Input: part model. Units: mm. Frame: model coordinates. A direction names the side the tool comes from. Coordinates: 2 decimals unless noted, no trailing zeros. Loops run counter-clockwise (first coordinate to the right, second up) from the corner with the lowest first, then second, coordinate; pieces in that order, holes last. Notation, with made-up numbers: (-17, 17) - (-5, 17) arc R20 ccw to (-5, 40) - close; hole circle Ø8 at (22.25, 9.25). An arc over 180 degrees is marked (long way). Use one line per item in the form item = value.
from build123d import *

# Parameters (mm, degrees)
SKETCH1_R           = 2.5
SKETCH1_R_2         = 3.5
SKETCH1_W           = 71.85
SKETCH1_H           = 24.6
SKETCH1_W_2         = 12.2
SKETCH1_H_2         = 12.2
SKETCH1_W_3         = 10.2
SKETCH1_H_3         = 14.85
BOSS_EXTRUDE1_DEPTH = 3
FILLET1_R           = 2
FILLET2_R           = 3
BOSS_EXTRUDE2_START = -10
BOSS_EXTRUDE2_DEPTH = 10
BOSS_EXTRUDE3_START = -10
BOSS_EXTRUDE3_DEPTH = 10


with BuildPart() as part:
    # Sketch1 → Boss-Extrude1 (new body)
    with BuildSketch(Plane.XY):
        Polygon((0, 0), (-115, 0), (-115, -51), (-143, -51), (-143, -99), (-115, -99), (0, -99), (28, -99), (28, -51), (0, -51), align=None)
        with Locations((-57.5, -10.395373235)):
            Circle(SKETCH1_R, mode=Mode.SUBTRACT)
        with Locations((-19.5, -32.493549158)):
            Circle(SKETCH1_R_2, mode=Mode.SUBTRACT)
        with Locations((-45.247302804, -78.7)):
            Rectangle(SKETCH1_W, SKETCH1_H, mode=Mode.SUBTRACT)
        with Locations((-98.6, -53.697377152)):
            Rectangle(SKETCH1_W_2, SKETCH1_H_2, mode=Mode.SUBTRACT)
        with Locations((-95.5, -32.493549158)):
            Rectangle(SKETCH1_W_3, SKETCH1_H_3, mode=Mode.SUBTRACT)
        with Locations((-16.4, -53.697377152)):
            Rectangle(SKETCH1_W_2, SKETCH1_H_2, mode=Mode.SUBTRACT)
    extrude(amount=BOSS_EXTRUDE1_DEPTH)

    # Fillet1
    fillet1_edges = [part.edges().sort_by_distance(p)[0] for p in [
        (-115, -25.5, 3),
        (-129, -51, 3),
        (-143, -75, 3),
        (-57.5, -99, 3),
        (28, -75, 3),
        (14, -51, 3),
        (0, -25.5, 3),
        (-57.5, 0, 3),
    ]]
    fillet(fillet1_edges, radius=FILLET1_R)

    # Fillet2
    # the kernel refuses this fillet: 3 mm, written as the material it takes off along each edge
    with BuildSketch(Plane(origin=(-140, -54, 3), x_dir=(0, 1, 0), z_dir=(1, 0, 0))) as fillet2_piece_1:
        with BuildLine():
            CenterArc((1, -2), 2, 0, 90)
            Line((3, -2), (3, 0))
            Line((3, 0), (1, 0))
        make_face()
    revolve(axis=Axis((-140, -54, 3), (0, 0, 1)), revolution_arc=90, mode=Mode.SUBTRACT)
    with BuildSketch(Plane(origin=(-140, -96, 3), x_dir=(-1, 0, 0), z_dir=(0, 1, 0))) as fillet2_piece_2:
        with BuildLine():
            CenterArc((1, -2), 2, 0, 90)
            Line((3, -2), (3, 0))
            Line((3, 0), (1, 0))
        make_face()
    revolve(axis=Axis((-140, -96, 3), (0, 0, 1)), revolution_arc=90, mode=Mode.SUBTRACT)
    with BuildSketch(Plane(origin=(-112, -3, 3), x_dir=(0, 1, 0), z_dir=(1, 0, 0))) as fillet2_piece_3:
        with BuildLine():
            CenterArc((1, -2), 2, 0, 90)
            Line((3, -2), (3, 0))
            Line((3, 0), (1, 0))
        make_face()
    revolve(axis=Axis((-112, -3, 3), (0, 0, 1)), revolution_arc=90, mode=Mode.SUBTRACT)
    with BuildSketch(Plane(origin=(25, -96, 3), x_dir=(0, -1, 0), z_dir=(-1, 0, 0))) as fillet2_piece_4:
        with BuildLine():
            CenterArc((1, -2), 2, 0, 90)
            Line((3, -2), (3, 0))
            Line((3, 0), (1, 0))
        make_face()
    revolve(axis=Axis((25, -96, 3), (0, 0, 1)), revolution_arc=90, mode=Mode.SUBTRACT)
    with BuildSketch(Plane(origin=(-3, -3, 3), x_dir=(1, 0, 0), z_dir=(0, -1, 0))) as fillet2_piece_5:
        with BuildLine():
            CenterArc((1, -2), 2, 0, 90)
            Line((3, -2), (3, 0))
            Line((3, 0), (1, 0))
        make_face()
    revolve(axis=Axis((-3, -3, 3), (0, 0, 1)), revolution_arc=90, mode=Mode.SUBTRACT)
    with BuildSketch(Plane(origin=(25, -54, 3), x_dir=(1, 0, 0), z_dir=(0, -1, 0))) as fillet2_piece_6:
        with BuildLine():
            CenterArc((1, -2), 2, 0, 90)
            Line((3, -2), (3, 0))
            Line((3, 0), (1, 0))
        make_face()
    revolve(axis=Axis((25, -54, 3), (0, 0, 1)), revolution_arc=90, mode=Mode.SUBTRACT)
    with BuildSketch(Plane(origin=(28, -51, -7.5), x_dir=(-1, 0, 0), z_dir=(0, 0, 1)), Plane(origin=(0, 0, -7.5), x_dir=(-1, 0, 0), z_dir=(0, 0, 1))) as fillet2_piece_7:
        with BuildLine():
            CenterArc((FILLET2_R, FILLET2_R), FILLET2_R, 180, 90)
            Line((0, FILLET2_R), (0, 0))
            Line((0, 0), (FILLET2_R, 0))
        make_face()
    extrude(amount=10.5, mode=Mode.SUBTRACT)
    with BuildSketch(Plane(origin=(-115, 0, -7.5), x_dir=(1, 0, 0), z_dir=(0, 0, 1)), Plane(origin=(-143, -51, -7.5), x_dir=(1, 0, 0), z_dir=(0, 0, 1)), Plane(origin=(28, -99, -7.5), x_dir=(-1, 0, 0), z_dir=(0, 0, 1)), Plane(origin=(-143, -99, -7.5), x_dir=(0, 1, 0), z_dir=(0, 0, 1))) as fillet2_piece_8:
        with BuildLine():
            CenterArc((FILLET2_R, -FILLET2_R), FILLET2_R, 90, 90)
            Line((0, -FILLET2_R), (0, 0))
            Line((0, 0), (FILLET2_R, 0))
        make_face()
    extrude(amount=10.5, mode=Mode.SUBTRACT)

    # Sketch3 → Boss-Extrude2 (add)
    with BuildSketch(Plane(origin=(0, -60, 0), x_dir=(1, 0, 0), z_dir=(0, 1, 0)).offset(BOSS_EXTRUDE2_START)):
        Polygon((25, 0), (25, 20), (26.5, 21.5), (26.5, 23.5), (22.525, 23.5), (19, 0), align=None)
        Polygon((-134, 0), (-140, 0), (-140, 20), (-141.5, 21.5), (-141.5, 23.5), (-137.525, 23.5), align=None)
    extrude(amount=-BOSS_EXTRUDE2_DEPTH)

    # Sketch4 → Boss-Extrude3 (add)
    with BuildSketch(Plane(origin=(0, 0, 0), x_dir=(1, 0, 0), z_dir=(0, 1, 0)).offset(BOSS_EXTRUDE3_START)):
        Polygon((-112, 0), (-106, 0), (-109.525, 23.5), (-113.5, 23.5), (-113.5, 21.5), (-112, 20), align=None)
        Polygon((-1.5, 21.5), (-1.5, 23.5), (-5.475, 23.5), (-9, 0), (-3, 0), (-3, 20), align=None)
    extrude(amount=-BOSS_EXTRUDE3_DEPTH)


solid = part.part
Q1. Cut plane A-A, the plane x = -19.5. Return loops of the section in (y, z).
Check values:
outline = (-99, 0) - (-91, 0) - (-91, 3) - (-97, 3) arc R2 ccw to (-99, 1) - close; (-66.4, 0) - (-59.8, 0) - (-59.8, 3) - (-66.4, 3) - close; (-47.6, 0) - (-35.99, 0) - (-35.99, 3) - (-47.6, 3) - close; (-28.99, 0) - (0, 0) - (0, 1) arc R2 ccw to (-2, 3) - (-28.99, 3) - close
Q2. Ray query, line 1 along Y through (x, z) = (-19.5, 1); line 2 along Y through (x, z) = (-57.5, 1); line 3 along Y through (x, z) = (-57.5, 1.75). Return the intervals inside material, ascending. Write a range as [from, to].
Check values:
line_1 = [-99, -91], [-66.4, -59.8], [-47.6, -35.99], [-28.99, 0]
line_2 = [-99, -91], [-66.4, -12.9], [-7.9, 0]
line_3 = [-98.85, -91], [-66.4, -12.9], [-7.9, -0.15]
Q3. Cut plane C-C, the plane x = -57.5. Return loops of the section in (y, z), then the cut area to 3 significant figures.
Check values:
outline = (-99, 0) - (-91, 0) - (-91, 3) - (-97, 3) arc R2 ccw to (-99, 1) - close; (-66.4, 0) - (-12.9, 0) - (-12.9, 3) - (-66.4, 3) - close; (-7.9, 0) - (0, 0) - (0, 1) arc R2 ccw to (-2, 3) - (-7.9, 3) - close
area = 206 mm²
Q4. Pull-direction query (Y, two-part tool) for faces 1 (the cylindrical face through (-0.86, -0.9, 0.49)), 2 (the flat face through (-138, -80, -12)), 3 (the flat face through (-9.322, -79, 1)); classes: pulls with the +Y half, pulls with the -Y half, needs draft (parallel to the pull), parting line crosses it, or undercut.
Check values:
face_1 = pulls with the +Y half
face_2 = pulls with the -Y half
face_3 = undercut
Q5. Set-up query: faces 4 (the flat face through (-140, -75, -10)), 5 (the flat face through (-46, -91, 1)), 6 (the flat face through (-110, -10, -12)), 7 (the flat face through (-135.787, -74.93, -11.914)), 8 (the cylindrical face through (27.1, -98.14, 0.49)). Return all of +Z, -Z, +X, -X, +Y, -Y with unobstructed straight access to the full face (end or side cutting, diameter ignored); none if empty.
Check values:
face_4 = -X, +Y, -Y
face_5 = +Z, -Z
face_6 = -Z, +X, -X, +Y
face_7 = -Z, +Y, -Y
face_8 = +Z, -Z, +X, -Y
Q6. First-contact query: P1, Ø10, axis at y = -66.5, z = -19.5, coming from the +X side; P2, Ø1.5, axis at x = -18, z = 2, coming from the +Y side; P3, Ø1.5, axis at y = -51.5, z = 2, coming from the +X side. Flat tips, straight axial feed; report the tip coordinate or a pass-through.
Check values:
P1 = 26.5
P2 = -0.02
P3 = 27.23
Q7. Cut plane B-B, the plane z = -14. Return loops of the section in (x, y), then the cut area to 3 significant figures.
Check values:
outline = (-140, -80) - (-136.1, -80) - (-136.1, -70) - (-140, -70) - close; (-112, -20) - (-108.1, -20) - (-108.1, -10) - (-112, -10) - close; (-6.9, -20) - (-3, -20) - (-3, -10) - (-6.9, -10) - close; (21.1, -80) - (25, -80) - (25, -70) - (21.1, -70) - close
area = 156 mm²
